```python
from build123d import *

# Parameters (mm, degrees)
BOSS_EXTRUDE1_DEPTH = 1.016
CUT_EXTRUDE1_START  = -0.635
CUT_EXTRUDE1_DEPTH  = 0.635
CUT_EXTRUDE2_DEPTH  = 19.211994839
CUT_EXTRUDE3_DEPTH  = 19.211994839


with BuildPart() as part:
    # Sketch1 → Boss-Extrude1 (new body)
    with BuildSketch(Plane.XY):
        with BuildLine():
            Line((-12.7, 7.62), (12.7, 7.62))
            ThreePointArc((12.7, 7.62), (15.394076836, 6.504076836), (16.51, 3.81))
            Line((16.51, 3.81), (16.51, 0))
            Line((16.51, 0), (-16.51, 0))
            Line((-16.51, 0), (-16.51, 3.81))
            ThreePointArc((-16.51, 3.81), (-15.394076836, 6.504076836), (-12.7, 7.62))
        make_face()
    extrude(amount=BOSS_EXTRUDE1_DEPTH)

    # Sketch2 → Cut-Extrude1 (cut)
    with BuildSketch(Plane.XY.offset(1.016).offset(CUT_EXTRUDE1_START)):
        with BuildLine():
            Line((16.2052, 0), (16.51, 0))
            Line((16.51, 0), (16.51, 3.81))
            ThreePointArc((16.51, 3.81), (15.394076836, 6.504076836), (12.7, 7.62))
            Line((12.7, 7.62), (-12.7, 7.62))
            ThreePointArc((-12.7, 7.62), (-15.394076836, 6.504076836), (-16.51, 3.81))
            Line((-16.51, 3.81), (-16.51, 0))
            Line((-16.51, 0), (-16.2052, 0))
            Line((-16.2052, 0), (-16.2052, 3.81))
            ThreePointArc((-16.2052, 3.81), (-15.178550689, 6.288550689), (-12.7, 7.3152))
            Line((-12.7, 7.3152), (12.7, 7.3152))
            ThreePointArc((12.7, 7.3152), (15.178550689, 6.288550689), (16.2052, 3.81))
            Line((16.2052, 3.81), (16.2052, 0))
        make_face()
    extrude(amount=CUT_EXTRUDE1_DEPTH, mode=Mode.SUBTRACT)

    # Sketch3 → Cut-Extrude2 (cut, through all)
    with BuildSketch(Plane.XY.offset(1.016)):
        with BuildLine():
            Line((-13.1826, 0), (-11.2446698, 1.9379302))
            ThreePointArc((-11.2446698, 1.9379302), (-10.4371152, 2.477520932), (-9.484539601, 2.667))
            Line((-9.484539601, 2.667), (9.484539601, 2.667))
            ThreePointArc((9.484539601, 2.667), (10.4371152, 2.477520932), (11.2446698, 1.9379302))
            Line((11.2446698, 1.9379302), (13.1826, 0))
            Line((13.1826, 0), (-13.1826, 0))
        make_face()
    extrude(amount=-CUT_EXTRUDE2_DEPTH, mode=Mode.SUBTRACT)

    # Sketch4 → Cut-Extrude3 (cut, through all)
    with BuildSketch(Plane.XY.offset(1.016)):
        with BuildLine():
            Line((16.51, 0), (15.24, 0))
            Line((15.24, 0), (15.24, 0.381))
            ThreePointArc((15.24, 0.381), (15.351592316, 0.650407684), (15.621, 0.762))
            Line((15.621, 0.762), (16.51, 0.762))
            Line((16.51, 0.762), (16.51, 0))
        make_face()
    extrude(amount=-CUT_EXTRUDE3_DEPTH, mode=Mode.SUBTRACT)


solid = part.part
```
Part model, mm, in its own coordinate system. A direction names the side the tool comes from. Round coordinates to 2 decimals unless told otherwise and drop trailing zeros. Loops run counter-clockwise (first coordinate to the right, second up) from the corner with the lowest first, then second, coordinate; pieces in that order, holes last. Notation, with made-up numbers: (84.5, 33) -> (126.5, 33) arc R9 cw to (126.5, 47) -> close; hole circle Ø9 at (47, 89). An arc over 180 degrees is marked (long way). Use a Markdown table: item, result.
1) Pull direction X, two halves, no side cores. Call faces 4 (the flat face through (12.2, 0.98, 0.52)), 5 (the cylindrical face through (15.4, 6.5, 0.2)), 6 (the cylindrical face through (-15.4, 6.5, 0.2)): pulls with the +X half, pulls with the -X half, needs draft (parallel to the pull), parting line crosses it, or undercut.
The answers:
| item | result |
|---|---|
| face 4 | undercut |
| face 5 | pulls with the +X half |
| face 6 | pulls with the -X half |
2) Cut at B-B, the plane y = 7. List the corners of the cut face in (x, z), and give its area (3 significant figures).
The answers:
| item | result |
|---|---|
| outline | (-14.78, 0) -> (14.78, 0) -> (14.78, 0.38) -> (14.15, 0.38) -> (14.15, 1.02) -> (-14.15, 1.02) -> (-14.15, 0.38) -> (-14.78, 0.38) -> close |
| area | 29.2 mm2 |
3) Cut at D-D, the plane x = 14.5. List the corners of the cut face in (y, z), and give its area (3 significant figures).
The answers:
| item | result |
|---|---|
| outline | (0, 0) -> (7.17, 0) -> (7.17, 0.38) -> (6.82, 0.38) -> (6.82, 1.02) -> (0, 1.02) -> close |
| area | 7.06 mm2 |
4) Cut at A-A, the plane z = 0.85. List the corners of the cut face in (x, y).
The answers:
| item | result |
|---|---|
| outline | (-16.21, 0) -> (-13.18, 0) -> (-11.24, 1.94) arc R2.49 cw to (-9.48, 2.67) -> (9.48, 2.67) arc R2.49 cw to (11.24, 1.94) -> (13.18, 0) -> (15.24, 0) -> (15.24, 0.38) arc R0.38 cw to (15.62, 0.76) -> (16.21, 0.76) -> (16.21, 3.81) arc R3.51 ccw to (12.7, 7.32) -> (-12.7, 7.32) arc R3.51 ccw to (-16.21, 3.81) -> close |
5) Probe line 1 (Y direction, x = 1.5, z = 0.1); line 2 (Y direction, x = -7, z = 0.45); line 3 (X direction, y = 2, z = 0.65). List the from-to ranges inside material, lowest first. Write a range as [from, to].
The answers:
| item | result |
|---|---|
| line 1 | y = [2.67, 7.62] |
| line 2 | y = [2.67, 7.32] |
| line 3 | x = [-16.21, -11.18], [11.18, 16.21] |
6) Drop a flat-ended pin along its axis: pin 1 Ø0.5 at (y, z) = (2.5, 1) entering from -X. Give the stop position or say it passes through.
The answers:
| item | result |
|---|---|
| pin 1 | stops at x = -16.21 |
7) Tool access for faces 1 (the cylindrical face through (15.151, 6.316, 0.694)), 2 (the cylindrical face through (-10.45, 2.47, 0.52)), 3 (the flat face through (16, 0.762, 0.5)): list every direction of +Z, -Z, +X, -X, +Y, -Y with a clear straight run to the whole face (end or side of a thin tool).
The answers:
| item | result |
|---|---|
| face 1 | +Z, +X, +Y |
| face 2 | +Z, -Z, -Y |
| face 3 | +Z, -Z, +X, -Y |
8) Cut at C-C, the plane x = -6. List the corners of the cut face in (y, z), and give its area (3 significant figures).
The answers:
| item | result |
|---|---|
| outline | (2.67, 0) -> (7.62, 0) -> (7.62, 0.38) -> (7.32, 0.38) -> (7.32, 1.02) -> (2.67, 1.02) -> close |
| area | 4.84 mm2 |
